CAD build for the part. Positions are in the model's coordinates, mm. Coordinates: 2 decimals unless noted, no trailing zeros. Order: outer loops, then holes, each group sorted by start corner. A loop starts at its lowest first (then second) coordinate and runs counter-clockwise, first axis right, second up. Notation, with made-up numbers: (73, -30.5) -> (92, -30.5) arc R25 ccw to (92, 2.5) -> close; hole circle Ø2 at (81, -33). An arc over 180 degrees is marked (long way). Use one line per item in the form item = value. Start each with the question number.
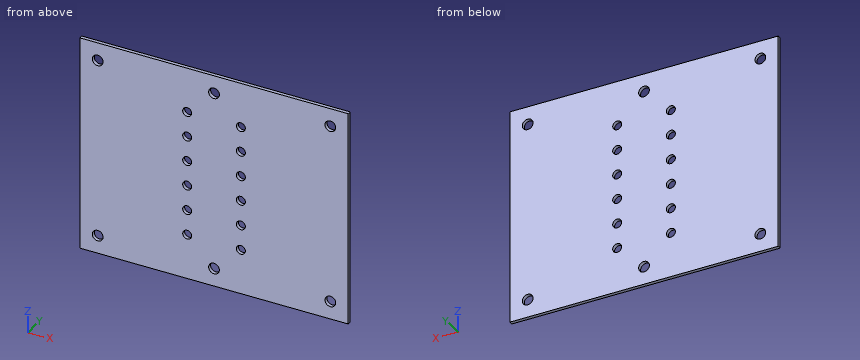
from build123d import *

# Parameters (mm, degrees)
SKETCH_1_W          = 75
SKETCH_1_H          = 60
EXTRUDE_1_DEPTH     = 1
SKETCH_2_R          = 1.25
CUT_EXTRUDE_1_DEPTH = 49.033842236
SKETCH_3_R          = 1.5
CUT_EXTRUDE_2_DEPTH = 49.033842236


with BuildPart() as part:
    # 草图1 → 凸台-拉伸1 (new body)
    with BuildSketch(Plane(origin=(0, 0, 0), x_dir=(1, 0, 0), z_dir=(0, 1, 0))):
        Rectangle(SKETCH_1_W, SKETCH_1_H)
    extrude(amount=EXTRUDE_1_DEPTH)

    # 草图2 → 切除-拉伸1 (cut, through all)
    with BuildSketch(Plane(origin=(0, 0, 0), x_dir=(1, 0, 0), z_dir=(0, 1, 0))):
        with Locations(Location((-7.5, 17.5, 0), (0, 0, 270))):
            Circle(SKETCH_2_R)
        with Locations(Location((7.5, 17.5, 0), (0, 0, 270))):
            Circle(SKETCH_2_R)
        with Locations(Location((7.5, 10.5, 0), (0, 0, 270))):
            Circle(SKETCH_2_R)
        with Locations(Location((7.5, 3.5, 0), (0, 0, 270))):
            Circle(SKETCH_2_R)
        with Locations(Location((7.5, -3.5, 0), (0, 0, 270))):
            Circle(SKETCH_2_R)
        with Locations(Location((7.5, -10.5, 0), (0, 0, 270))):
            Circle(SKETCH_2_R)
        with Locations(Location((7.5, -17.5, 0), (0, 0, 270))):
            Circle(SKETCH_2_R)
        with Locations(Location((-7.5, 10.5, 0), (0, 0, 270))):
            Circle(SKETCH_2_R)
        with Locations(Location((-7.5, 3.5, 0), (0, 0, 270))):
            Circle(SKETCH_2_R)
        with Locations(Location((-7.5, -3.5, 0), (0, 0, 270))):
            Circle(SKETCH_2_R)
        with Locations(Location((-7.5, -10.5, 0), (0, 0, 270))):
            Circle(SKETCH_2_R)
        with Locations(Location((-7.5, -17.5, 0), (0, 0, 270))):
            Circle(SKETCH_2_R)
    extrude(amount=CUT_EXTRUDE_1_DEPTH, mode=Mode.SUBTRACT)

    # 草图3 → 切除-拉伸2 (cut, through all)
    with BuildSketch(Plane(origin=(0, 0, 0), x_dir=(1, 0, 0), z_dir=(0, 1, 0))):
        with Locations(Location((-32.5, 25, 0), (0, 0, 270))):
            Circle(SKETCH_3_R)
        with Locations(Location((32.5, -25, 0), (0, 0, 270))):
            Circle(SKETCH_3_R)
        with Locations(Location((-32.5, -25, 0), (0, 0, 90))):
            Circle(SKETCH_3_R)
        with Locations(Location((32.5, 25, 0), (0, 0, 90))):
            Circle(SKETCH_3_R)
        with Locations(Location((0, -25, 0), (0, 0, 90))):
            Circle(SKETCH_3_R)
        with Locations(Location((0, 25, 0), (0, 0, 270))):
            Circle(SKETCH_3_R)
    extrude(amount=CUT_EXTRUDE_2_DEPTH, mode=Mode.SUBTRACT)


solid = part.part
1) Cut at B-B on z = -25. Give the cut face in (x, y), then the cut area to 3 significant figures.
2) Probe L1, parallel to Z at x = 32.5, y = 0.3; L2, parallel to X at y = 0.55, z = -25; L3, parallel to X at y = 0.65, z = -10.5. List the from-to ranges inside material, lowest first.
3) Cut at A-A on x = -7.5. Give the cut face in (y, z).
4) Cut at C-C on y = 0.2. Count the separate pieces of the cut face and the enclosed holes in it, then the cut area to 3 significant figures.
5) Cut at D-D on z = -10.5. Give the cut face in (x, y), then the cut area to 3 significant figures.
6) Drop a flat-ended pin along its axis: P1, Ø2, axis at x = -7.5, z = -10.5, coming from the -Y side. Give the stop position or say it passes through.
Values follow:
q1.outline = (-37.5, 0) -> (-34, 0) -> (-34, 1) -> (-37.5, 1) -> close; (-31, 0) -> (-1.5, 0) -> (-1.5, 1) -> (-31, 1) -> close; (1.5, 0) -> (31, 0) -> (31, 1) -> (1.5, 1) -> close; (34, 0) -> (37.5, 0) -> (37.5, 1) -> (34, 1) -> close
q1.area = 66.0 mm^2
q2.L1 = -30 to -26.5, -23.5 to 23.5, 26.5 to 30
q2.L2 = -37.5 to -34, -31 to -1.5, 1.5 to 31, 34 to 37.5
q2.L3 = -37.5 to -8.75, -6.25 to 6.25, 8.75 to 37.5
q3.outline = (0, -30) -> (1, -30) -> (1, -18.75) -> (0, -18.75) -> close; (0, -16.25) -> (1, -16.25) -> (1, -11.75) -> (0, -11.75) -> close; (0, -9.25) -> (1, -9.25) -> (1, -4.75) -> (0, -4.75) -> close; (0, -2.25) -> (1, -2.25) -> (1, 2.25) -> (0, 2.25) -> close; (0, 4.75) -> (1, 4.75) -> (1, 9.25) -> (0, 9.25) -> close; (0, 11.75) -> (1, 11.75) -> (1, 16.25) -> (0, 16.25) -> close; (0, 18.75) -> (1, 18.75) -> (1, 30) -> (0, 30) -> close
q4.separate_pieces = 1
q4.enclosed_holes = 18
q4.area = 4,400 mm^2
q5.outline = (-37.5, 0) -> (-8.75, 0) -> (-8.75, 1) -> (-37.5, 1) -> close; (-6.25, 0) -> (6.25, 0) -> (6.25, 1) -> (-6.25, 1) -> close; (8.75, 0) -> (37.5, 0) -> (37.5, 1) -> (8.75, 1) -> close
q5.area = 70.0 mm^2
q6.P1 = through
